```python
from build123d import *

# Parameters (mm, degrees)
F0_R     = 0.5
F1_DEPTH = 3
F2_DEPTH = 10


with BuildPart() as f1:
    # F0 (on Top) → F1 (new body)
    with BuildSketch(Plane.XY):
        with BuildLine():
            ThreePointArc((0, -6.5), (4.596194, -4.596194), (6.5, 0))
            ThreePointArc((6.5, 0), (4.596194, 4.596194), (0, 6.5))
            ThreePointArc((0, 6.5), (-6.5, 0), (0, -6.5))
        make_face()
        with BuildLine():
            ThreePointArc((2, 1.5), (2.5, 0), (2, -1.5))
            Line((2, -1.5), (-2, -1.5))
            ThreePointArc((-2, -1.5), (-2.5, 0), (-2, 1.5))
            Line((-2, 1.5), (2, 1.5))
        make_face(mode=Mode.SUBTRACT)
        with BuildLine():
            ThreePointArc((0, 6.5), (4.596194, 4.596194), (6.5, 0))
            ThreePointArc((6.5, 0), (4.596194, -4.596194), (0, -6.5))
            Line((0, -6.5), (30, -6.5))
            ThreePointArc((30, -6.5), (23.5, 0), (30, 6.5))
            Line((30, 6.5), (0, 6.5))
        make_face()
        with BuildLine():
            ThreePointArc((36.5, 0), (34.596194, 4.596194), (30, 6.5))
            ThreePointArc((30, 6.5), (23.5, 0), (30, -6.5))
            ThreePointArc((30, -6.5), (34.596194, -4.596194), (36.5, 0))
        make_face()
        with Locations((30, 0)):
            Circle(F0_R, mode=Mode.SUBTRACT)
    extrude(amount=F1_DEPTH)

    # F0 (on Top) → F2 (join)
    with BuildSketch(Plane.XY):
        with BuildLine():
            ThreePointArc((0, -6.5), (4.596194, -4.596194), (6.5, 0))
            ThreePointArc((6.5, 0), (4.596194, 4.596194), (0, 6.5))
            ThreePointArc((0, 6.5), (-6.5, 0), (0, -6.5))
        make_face()
        with BuildLine():
            ThreePointArc((2, 1.5), (2.5, 0), (2, -1.5))
            Line((2, -1.5), (-2, -1.5))
            ThreePointArc((-2, -1.5), (-2.5, 0), (-2, 1.5))
            Line((-2, 1.5), (2, 1.5))
        make_face(mode=Mode.SUBTRACT)
    extrude(amount=-F2_DEPTH)


solid = f1.part
```
Geometry: final body of the model. Coordinates: model frame, mm. A direction names the side the tool comes from. Round coordinates to 2 decimals unless told otherwise and drop trailing zeros. Order: outer loops, then holes, each group sorted by start corner. A loop starts at its lowest first (then second) coordinate and runs counter-clockwise, first axis right, second up. Notation, with made-up numbers: M 62.5,3.25 L 75.5,3.25 A27 ccw 75.5,19.25 Z; hole C 86,44 d8. An arc over 180 degrees is marked long. One line per item, written item: value.
(1) Cut plane C-C (x = 12). Return the cut outline in (y, z).
Result sheet:
outline: M -6.5,0 L 6.5,0 L 6.5,3 L -6.5,3 Z
(2) Cut plane B-B (z = -3.25). Return the cut outline in (x, y).
Result sheet:
outline: C 0,0 d13; hole M -2,-1.5 L 2,-1.5 A2.5 ccw 2,1.5 L -2,1.5 A2.5 ccw Z
(3) Cut plane D-D (y = 5.75). Return the cut outline in (x, z).
Result sheet:
outline: M -3.03,-10 L 3.03,-10 L 3.03,0 L 33.03,0 L 33.03,3 L -3.03,3 Z
(4) Cut plane A-A (y = 1). Return the cut outline in (x, z), and give its area (3 significant figures).
Result sheet:
outline: M -6.42,-10 L -2.29,-10 L -2.29,3 L -6.42,3 Z; M 2.29,-10 L 6.42,-10 L 6.42,0 L 36.42,0 L 36.42,3 L 2.29,3 Z
area: 197 mm2
(5) Reachability of faces 3 (the flat face through (15, 6.5, 1)), 4 (the flat face through (0, 1.5, -3)) from +Z, -Z, +X, -X, +Y, -Y: full face, straight path, thin tool, end or side. Return the list, or none.
Result sheet:
face 3: +Z, -Z, +X, -X, +Y
face 4: +Z, -Z
(6) Line query: probe 1 along Y at (x, z) = (30, 1.05); probe 2 along Z at (x, y) = (23, 5.75); probe 3 along X at (y, z) = (-0.5, -2.25). Output: solid intervals per line, ascending. Write a range as [from, to].
Result sheet:
probe 1: [-6.5, -0.5], [0.5, 6.5]
probe 2: [0, 3]
probe 3: [-6.48, -2.45], [2.45, 6.48]
(7) Pin query (flat end, axial travel): P1, Ø4, axis at x = 12.5, z = -1, coming from the -Y side; P2, Ø1.5, axis at x = 21, y = 2, coming from the -Z side. Return the tip coordinate at first contact, or that it passes through.
Result sheet:
P1: y = -6.5
P2: z = 0
(8) Pull-direction query (X, two-part tool) for faces 1 (the flat face through (15, 0, 3)), 2 (the flat face through (0, -1.5, -3)); classes: pulls with the +X half, pulls with the -X half, needs draft (parallel to the pull), parting line crosses it, or undercut.
Result sheet:
face 1: needs draft
face 2: undercut
